Geometry check sheet. Reference: the model listing, model coordinates, mm. Face numbers are marked on the shaded views. A direction names the side the tool comes from. Give positions to 0.01 mm unless a question says otherwise; leave off trailing zeros. Write each loop counter-clockwise with the first axis right and the second up, starting at its lowest first coordinate (ties: lowest second). Pieces come first, ordered by that corner, then holes. Notation, with made-up numbers: (-21.5, -9.5) -> (-14.5, -9.5) arc R18 ccw to (-14.5, 16.5) -> close; hole circle Ø3 at (-34.75, 85.25). An arc over 180 degrees is marked (long way). Write item = value, one per line. Start each with the question number.
1. Set-up check for the marked faces 4, 5 and 6: record each of +Z, -Z, +X, -X, +Y, -Y from which the full face is reachable in a straight line by a thin tool's end or side.
2. Cross-section at C-C, the plane y = -10.25. Record the cut outline in (x, z), plus the area to 3 significant figures.
3. Mould release check, pull along X, two halves, no side actions. Record for the marked faces 1, 2 and 3: pulls with the +X half, pulls with the -X half, needs draft (parallel to the pull), parting line crosses it, or undercut.
4. Depth check by flat-ended pin: P1, Ø4, axis at x = -31.44, z = 17.5, coming from the -Y side; P2, Ø1.5, axis at y = 1, z = 13.5, coming from the -X side; P3, Ø2.5, axis at x = -31.44, z = 17.5, coming from the -Y side; P4, Ø3, axis at x = -32, y = 2, coming from the -Z side. Enter the tip coordinate at first touch or a pass-through.
5. Thickness scan on line 1 along X through (y, z) = (0.5, 7.5); line 2 along X through (y, z) = (-2, 5.25); line 3 along Z through (x, y) = (-5, -10.5). Record the ranges inside material, lowest first.
6. Cross-section at B-B, the plane z = 1.75. Record the cut outline in (x, y) (3 decimals), plus the area to 3 significant figures.
7. Cross-section at A-A, the plane x = 2.5. Record the cut outline in (y, z).
8. Cross-section at D-D, the plane z = 17.5. Record the cut outline in (x, y), plus the area to 3 significant figures.
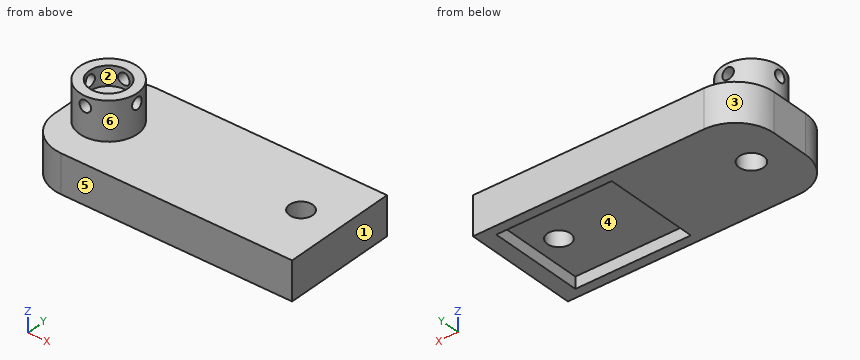
```python
from build123d import *

# Parameters (mm, degrees)
BOSS_EXTRUDE1_DEPTH             = 10
SKETCH6_W                       = 30
SKETCH6_H                       = 25
CUT_EXTRUDE1_DEPTH              = 3
SKETCH8_R                       = 3
CUT_EXTRUDE2_DEPTH              = 10
SKETCH9_R                       = 7.5
BOSS_EXTRUDE2_DEPTH             = 10
SKETCH10_R                      = 5
CUT_EXTRUDE3_DEPTH              = 5
SKETCH11_R                      = 1.5
CUT_EXTRUDE4_DEPTH              = 49.621106648
CIRPATTERN1_COUNT               = 2
CIRPATTERN1_ANGLE               = 90
F_1_4_0_25_DIAMETER_HOLE1_D     = 6.35
F_1_4_0_25_DIAMETER_HOLE1_DEPTH = 10
F_1_4_0_25_DIAMETER_HOLE1_TIP   = 1.907732465


with BuildPart() as part:
    # Sketch1 → Boss-Extrude1 (new body)
    with BuildSketch(Plane.XY):
        with BuildLine():
            Line((-41.436145974, 5.718072987), (-41.436145974, -4.281927013))
            ThreePointArc((-41.436145974, -4.281927013), (-38.507213786, -11.352994825), (-31.436145974, -14.281927013))
            Line((-31.436145974, -14.281927013), (28.563854026, -14.281927013))
            Line((28.563854026, -14.281927013), (28.563854026, 15.718072987))
            Line((28.563854026, 15.718072987), (-31.436145974, 15.718072987))
            ThreePointArc((-31.436145974, 15.718072987), (-38.507213786, 12.789140799), (-41.436145974, 5.718072987))
        make_face()
    extrude(amount=BOSS_EXTRUDE1_DEPTH)

    # Sketch6 → Cut-Extrude1 (cut)
    with BuildSketch(Plane(origin=(0, 0, 0), x_dir=(-1, 0, 0), z_dir=(0, 0, -1))):
        with Locations((-9.563854026, 0.718072987)):
            Rectangle(SKETCH6_W, SKETCH6_H)
    extrude(amount=-CUT_EXTRUDE1_DEPTH, mode=Mode.SUBTRACT)

    # Sketch8 → Cut-Extrude2 (cut)
    with BuildSketch(Plane.XY.offset(10)):
        with Locations((18.563854026, 0.718072987)):
            Circle(SKETCH8_R)
    extrude(amount=-CUT_EXTRUDE2_DEPTH, mode=Mode.SUBTRACT)

    # Sketch9 → Boss-Extrude2 (add)
    with BuildSketch(Plane.XY.offset(10)):
        with Locations((-31.436145974, 0.718072987)):
            Circle(SKETCH9_R)
    extrude(amount=BOSS_EXTRUDE2_DEPTH)

    # Sketch10 → Cut-Extrude3 (cut)
    with BuildSketch(Plane.XY.offset(20)):
        with Locations((-31.436145974, 0.718072987)):
            Circle(SKETCH10_R)
    extrude(amount=-CUT_EXTRUDE3_DEPTH, mode=Mode.SUBTRACT)

    # Sketch11 → Cut-Extrude4 (cut, symmetric)
    with BuildSketch(Plane(origin=(0, 0, 0), x_dir=(1, 0, 0), z_dir=(0, 1, 0))):
        with Locations(Location((-31.436145974, -17.5, 0), (0, 0, 270))):
            Circle(SKETCH11_R)
    cut_extrude4 = extrude(amount=CUT_EXTRUDE4_DEPTH, both=True, mode=Mode.SUBTRACT)

    # CirPattern1: Cut-Extrude4 ×2 about axis
    cirpattern1_axis = Axis((-31.436145974, 0.718072987, 20), (0, 0, -1))
    for i in range(1, CIRPATTERN1_COUNT):
        add(cut_extrude4.rotate(cirpattern1_axis, i * CIRPATTERN1_ANGLE / (CIRPATTERN1_COUNT - 1)), mode=Mode.SUBTRACT)

    # 1/4 (0.25) Diameter Hole1
    with Locations(Plane(origin=(0, 0, 0), x_dir=(-1, 0, 0), z_dir=(0, 0, -1))):
        with Locations((31.436145974, 0.718072987)):
            Hole(F_1_4_0_25_DIAMETER_HOLE1_D / 2, depth=F_1_4_0_25_DIAMETER_HOLE1_DEPTH)
            with Locations((0, 0, -(F_1_4_0_25_DIAMETER_HOLE1_DEPTH + F_1_4_0_25_DIAMETER_HOLE1_TIP / 2))):  # 118° drill point
                Cone(0, F_1_4_0_25_DIAMETER_HOLE1_D / 2, F_1_4_0_25_DIAMETER_HOLE1_TIP, mode=Mode.SUBTRACT)


solid = part.part
```
Answers:
q1.face_4 = -Z
q1.face_5 = +Z, -Z, +X, -X, -Y
q1.face_6 = +Z
q2.outline = (-39.46, 0) -> (-5.44, 0) -> (-5.44, 3) -> (24.56, 3) -> (24.56, 0) -> (28.56, 0) -> (28.56, 10) -> (-39.46, 10) -> close
q2.area = 590 mm^2
q3.face_1 = pulls with the +X half
q3.face_2 = undercut
q3.face_3 = pulls with the -X half
q4.P1 = -6.78
q4.P2 = -38.94
q4.P3 = through
q4.P4 = 10.16
q5.line_1 = -41.44 to -34.6, -28.27 to 15.57, 21.56 to 28.56
q5.line_2 = -41.44 to -33.08, -29.8 to 17.29, 19.83 to 28.56
q5.line_3 = 3 to 10
q6.outline = (-41.436, -4.282) arc R10 ccw to (-31.436, -14.282) -> (28.564, -14.282) -> (28.564, 15.718) -> (-31.436, 15.718) arc R10 ccw to (-41.436, 5.718) -> close; hole circle Ø6.35 at (-31.436, 0.718); hole (-5.436, -11.782) -> (24.564, -11.782) -> (24.564, 13.218) -> (-5.436, 13.218) -> close
q6.area = 1,280 mm^2
q7.outline = (-14.28, 0) -> (-11.78, 0) -> (-11.78, 3) -> (13.22, 3) -> (13.22, 0) -> (15.72, 0) -> (15.72, 10) -> (-14.28, 10) -> close
q8.outline = (-38.78, -0.78) arc R7.5 ccw to (-32.94, -6.63) -> (-32.94, -4.05) arc R5 cw to (-36.21, -0.78) -> close; (-38.78, 2.22) -> (-36.21, 2.22) arc R5 cw to (-32.94, 5.49) -> (-32.94, 8.07) arc R7.5 ccw to start; (-29.94, -6.63) arc R7.5 ccw to (-24.09, -0.78) -> (-26.67, -0.78) arc R5 cw to (-29.94, -4.05) -> close; (-29.94, 5.49) arc R5 cw to (-26.67, 2.22) -> (-24.09, 2.22) arc R7.5 ccw to (-29.94, 8.07) -> close
q8.area = 67.9 mm^2
